from build123d import *

# Parameters (mm, degrees)
F0_R     = 6
F1_DEPTH = 11.7
F4_SIZE  = 1


with BuildPart() as f1:
    # F0 (on Top) → F1 (new body)
    with BuildSketch(Plane.XY):
        Polygon((6.333883, 10.970607), (-6.333883, 10.970607), (-12.667766, 0), (-6.333883, -10.970607), (6.333883, -10.970607), (12.667766, 0), align=None)
        Circle(F0_R, mode=Mode.SUBTRACT)
    extrude(amount=F1_DEPTH)

    # F2 (on Right) → F3 (revolve, cut)
    with BuildSketch(Plane.YZ):
        Polygon((13.277913, 12.61499), (9.648551, 12.201084), (13.277913, 9.649714), align=None)
        Polygon((13.277913, 2.050286), (9.648551, -0.501084), (13.277913, -0.91499), align=None)
    revolve(axis=Axis((0, 0, 5.981519), (0, 0, -1)), mode=Mode.SUBTRACT)

    # F4
    f4_edges = [f1.edges().sort_by_distance(p)[0] for p in [
        (-6, 0, 11.7),
        (-6, 0, 0),
    ]]
    chamfer(f4_edges, length=F4_SIZE)


solid = f1.part
For this review, take the finished solid that the model builds, in its own axes (mm). Coordinates: 2 decimals unless noted, no trailing zeros. Order: outer loops, then holes, each group sorted by start corner. A loop starts at its lowest first (then second) coordinate and runs counter-clockwise, first axis right, second up. Notation, with made-up numbers: (81.5, 59) -> (120.5, 59) arc R21 ccw to (120.5, 97) -> close; hole circle Ø7 at (84, 86.25). An arc over 180 degrees is marked (long way). Return JSON: item names as keys, results as strings.
1. For pin 1 Ø1.5 at (y, z) = (2.5, 6.5) entering from +X; pin 2 Ø2 at (x, z) = (-7.5, 3.5) entering from -Y; pin 3 Ø9.5 at (x, y) = (0, 0) entering from -Z; pin 4 Ø5 at (y, z) = (-5.5, 2) entering from -X, all flat-tipped, find the tip position at first contact; note any pin that passes through.
Answer block:
{"pin 1": "x = 11.66", "pin 2": "y = -10.68", "pin 3": "through", "pin 4": "x = -10.94"}
2. The part is to be moulded in two halves that separate along Y. For faces 1 (the flat face through (9.46, -5.56, 5.77)), 2 (the cylindrical face through (-6, 0, 6)), 3 (the flat face through (2, -7, 0)), say which applies: +Y half, -Y half, draft (parallel to the pull), parting line (faces both ways), or undercut.
Answer block:
{"face 1": "-Y half", "face 2": "undercut", "face 3": "draft"}
3. We need section A-A on x = 0. Write out the cut boundary in (y, z).
Answer block:
{"outline": "(-10.97, 0.43) -> (-10.36, 0) -> (-7, 0) -> (-6, 1) -> (-6, 10.7) -> (-7, 11.7) -> (-10.36, 11.7) -> (-10.97, 11.27) -> close; (6, 1) -> (7, 0) -> (10.36, 0) -> (10.97, 0.43) -> (10.97, 11.27) -> (10.36, 11.7) -> (7, 11.7) -> (6, 10.7) -> close"}
4. We need section B-B on z = 5.25. Write out the cut boundary in (x, y), and give its area (3 significant figures).
Answer block:
{"outline": "(-12.67, 0) -> (-6.33, -10.97) -> (6.33, -10.97) -> (12.67, 0) -> (6.33, 10.97) -> (-6.33, 10.97) -> close; hole circle Ø12 at (0, 0)", "area": "304 mm²"}
5. For line 1 (Y direction, x = 0, z = 7); line 2 (Y direction, x = -4.5, z = 10); line 3 (X direction, y = -4.25, z = 9.5), list the stretches that pass through material, from the lowest coordinate up. Write a range as from..to.
Answer block:
{"line 1": "-10.97..-6, 6..10.97", "line 2": "-10.97..-3.97, 3.97..10.97", "line 3": "-10.21..-4.24, 4.24..10.21"}
